Here's how the part is built. I have some questions about the finished solid (model axes, mm). A direction names the side the tool comes from. Coordinates: 2 decimals unless noted, no trailing zeros. Write each loop counter-clockwise with the first axis right and the second up, starting at its lowest first coordinate (ties: lowest second). Pieces come first, ordered by that corner, then holes. Notation, with made-up numbers: (7.25, 50.5) - (54.25, 50.5) arc R22 ccw to (54.25, 64.5) - close; hole circle Ø3 at (22.25, -18). An arc over 180 degrees is marked (long way). Answer in a Markdown table with one row per item. Add a question column.
Item 1: I'm going to push flat-ended pins straight in: pin 1 (5 mm diameter, centred on x = 35, y = 10.5, fed in from +Z); pin 2 (2 mm diameter, centred on x = 15, y = 7, fed in from -Z); pin 3 (0.9 mm diameter, centred on y = 5, z = -7, fed in from +X); pin 4 (1.5 mm diameter, centred on x = 27, y = 5.5, fed in from -Z). Where does each tip first touch, or does it pass through?
Item 2: Imagine slicing it at B-B (x = 19.5). Please give me the cut outline in (y, z).
Item 3: If I drill on probe 1 along Y at (x, z) = (12, -3); probe 2 along Z at (x, y) = (11, 6.25); probe 3 along X at (y, z) = (1.75, -6), over which ranges is the centre line in solid material (lowest first)? Write a range as from..to.
Item 4: Imagine slicing it at D-D (x = 29). Please give me the cut outline in (y, z).
Item 5: We'd pull the mould along Y, two halves only. Please class faces 6 (the face through (14, 12, -5)), 7 (the face through (26, 2, -5.883)), 8 (the face through (16, 6, -2.765)), 9 (the face through (27.62, 0.94, -4.99)): +Y half, -Y half, draft (parallel to the pull), parting line (faces both ways), or undercut.
Item 6: Imagine slicing it at C-C (z = -5.5). Please give me the cut outline in (x, y).
Item 7: Imagine slicing it at A-A (y = 7.75). Please give me the cut outline in (x, z).
Item 8: Which directions (+Z, -Z, +X, -X, +Y, -Y) give clear straight access to the entire face, cutting with the end or side of a thin tool? Please do faces 1 (the face through (11, 6, -8.883)), 2 (the face through (11, 6, -6.443)), 3 (the face through (16, 9.736, -5)), 4 (the face through (27.62, 11.06, -4.99)), 5 (the face through (26, 10, -5.883)).
from build123d import *

# Parameters (mm, degrees)
BOSS_EXTRUDE1_DEPTH = 12
CUT_EXTRUDE1_DEPTH  = 8
CUT_EXTRUDE2_DEPTH  = 8
SKETCH6_W           = 4.5
SKETCH6_H           = 12
BOSS_EXTRUDE2_DEPTH = 3
BOSS_EXTRUDE3_DEPTH = 12
CUT_EXTRUDE3_START  = -14.451452
SKETCH8_W           = 3.67843884
SKETCH8_H           = 7.47183246
CUT_EXTRUDE3_DEPTH  = 14.451452


with BuildPart() as part:
    # Sketch1 → Boss-Extrude1 (new body)
    with BuildSketch(Plane(origin=(0, 0, 0), x_dir=(1, 0, 0), z_dir=(0, 1, 0))):
        Polygon((20.786387433, 2.157277486), (8.786387433, 2.157277486), (8.786387433, 5.883484052), (39.417420271, 5.883484052), align=None)
    extrude(amount=BOSS_EXTRUDE1_DEPTH)

    # Sketch4 → Cut-Extrude1 (cut)
    with BuildSketch(Plane(origin=(0, 0, -5.883484052), x_dir=(-1, 0, 0), z_dir=(0, 0, -1))):
        Polygon((-39.417420271, 3.299999999), (-22.917420271, 0), (-39.417420271, 0), align=None)
    cut_extrude1 = extrude(amount=-CUT_EXTRUDE1_DEPTH, mode=Mode.SUBTRACT)

    # Sketch5 → Cut-Extrude2 (cut)
    with BuildSketch(Plane(origin=(0, 0, -5.883484052), x_dir=(-1, 0, 0), z_dir=(0, 0, -1))):
        Polygon((-39.417420271, 6.5), (-23.237839122, 9.73591623), (-23.237839122, 2.26408377), (-39.417420271, 5.5), align=None)
    extrude(amount=-CUT_EXTRUDE2_DEPTH, mode=Mode.SUBTRACT)

    # Mirror1: Cut-Extrude1 across plane
    add(cut_extrude1.mirror(Plane.ZX.offset(6)), mode=Mode.SUBTRACT)

    # Sketch6 → Boss-Extrude2 (add)
    with BuildSketch(Plane(origin=(0, 0, -5.883484052), x_dir=(-1, 0, 0), z_dir=(0, 0, -1))):
        with Locations((-11.03638743, 6)):
            Rectangle(SKETCH6_W, SKETCH6_H)
    extrude(amount=BOSS_EXTRUDE2_DEPTH)

    # Sketch7 → Boss-Extrude3 (add)
    with BuildSketch(Plane(origin=(0, 12, 0), x_dir=(1, 0, 0), z_dir=(0, 1, 0))):
        Polygon((20.786387433, 2.157277486), (18.825226081, 1.765045216), (8.786387433, 1.765045216), (8.786387433, 2.157277486), align=None)
    extrude(amount=-BOSS_EXTRUDE3_DEPTH)

    # Sketch8 → Cut-Extrude3 (cut)
    with BuildSketch(Plane.ZY.offset(-8.786387433).offset(CUT_EXTRUDE3_START)):
        with Locations((-4.604264636, 6)):
            Rectangle(SKETCH8_W, SKETCH8_H)
    extrude(amount=CUT_EXTRUDE3_DEPTH, mode=Mode.SUBTRACT)


solid = part.part
Here are the results:
| question | item | result |
|---|---|---|
| 1 | pin 1 | stops at z = -4.51 |
| 1 | pin 2 | stops at z = -2.77 |
| 1 | pin 3 | stops at x = 13.29 |
| 1 | pin 4 | passes through |
| 2 | outline | (0, -5.88) - (2.26, -5.88) - (2.26, -2.77) - (9.74, -2.77) - (9.74, -5.88) - (12, -5.88) - (12, -1.9) - (0, -1.9) - close |
| 3 | probe 1 | y = 0..2.26, 9.74..12 |
| 3 | probe 2 | z = -8.88..-6.44, -2.77..-1.77 |
| 3 | probe 3 | x = 8.79..13.29 |
| 4 | outline | (1.22, -5.88) - (3.42, -5.88) - (3.42, -3.8) - (1.22, -3.8) - close; (8.58, -5.88) - (10.78, -5.88) - (10.78, -3.8) - (8.58, -3.8) - close |
| 5 | face 6 | +Y half |
| 5 | face 7 | draft |
| 5 | face 8 | undercut |
| 5 | face 9 | -Y half |
| 6 | outline | (8.79, 0) - (22.92, 0) - (37.5, 2.92) - (37.5, 5.12) - (23.24, 2.26) - (8.79, 2.26) - close; (8.79, 9.74) - (23.24, 9.74) - (37.5, 6.88) - (37.5, 9.08) - (22.92, 12) - (8.79, 12) - close |
| 7 | outline | (8.79, -8.88) - (13.29, -8.88) - (13.29, -6.44) - (8.79, -6.44) - close; (8.79, -2.77) - (23.24, -2.77) - (23.24, -2.65) - (18.83, -1.77) - (8.79, -1.77) - close; (33.17, -5.88) - (39.42, -5.88) - (33.17, -4.63) - close |
| 8 | face 1 | -Z, +X, -X, +Y, -Y |
| 8 | face 2 | +X, -X |
| 8 | face 3 | -X |
| 8 | face 4 | +Z, -Z, +X, +Y |
| 8 | face 5 | -Z, +X, +Y, -Y |
